from build123d import *

# Parameters (mm, degrees)
SKETCH1_W           = 18.56
SKETCH1_H           = 33.36
BOSS_EXTRUDE1_DEPTH = 1.64
FILLET1_R           = 1.2
SKETCH2_W           = 9.12
SKETCH2_H           = 5.3
CUT_EXTRUDE1_DEPTH  = 35.665510237
BOSS_EXTRUDE2_DEPTH = 6.1
SKETCH4_W           = 6.35
SKETCH4_H           = 0.5
CUT_EXTRUDE2_DEPTH  = 5
SKETCH5_W           = 6.35
SKETCH5_H           = 0.5
CUT_EXTRUDE3_DEPTH  = 0.4
SKETCH7_W           = 7
SKETCH7_H           = 7
BOSS_EXTRUDE3_DEPTH = 1.25
SKETCH8_W           = 3
SKETCH8_H           = 2.13
BOSS_EXTRUDE4_DEPTH = 1


with BuildPart() as part:
    # Sketch1 → Boss-Extrude1 (new body)
    with BuildSketch(Plane(origin=(0, 0, 0), x_dir=(1, 0, 0), z_dir=(0, 1, 0))):
        with Locations((0, -16.68)):
            Rectangle(SKETCH1_W, SKETCH1_H)
    extrude(amount=BOSS_EXTRUDE1_DEPTH)

    # Fillet1
    fillet1_edges = [part.edges().sort_by_distance(p)[0] for p in [
        (-9.28, 0.82, 0),
        (9.28, 0.82, 0),
        (9.28, 0.82, 33.36),
        (-9.28, 0.82, 33.36),
    ]]
    fillet(fillet1_edges, radius=FILLET1_R)

    # Sketch2 → Cut-Extrude1 (cut, through all)
    with BuildSketch(Plane(origin=(0, 1.64, 0), x_dir=(1, 0, 0), z_dir=(0, 1, 0))):
        with Locations((0, -2.65)):
            Rectangle(SKETCH2_W, SKETCH2_H)
    extrude(amount=-CUT_EXTRUDE1_DEPTH, mode=Mode.SUBTRACT)

    # Sketch3 → Boss-Extrude2 (add)
    with BuildSketch(Plane(origin=(0, 0, 5.3), x_dir=(-1, 0, 0), z_dir=(0, 0, -1))):
        with BuildLine():
            Line((-3.175, 0), (3.175, 0))
            ThreePointArc((3.175, 0), (4.094238816, 0.380761184), (4.475, 1.3))
            Line((4.475, 1.3), (4.475, 1.8))
            ThreePointArc((4.475, 1.8), (4.094238816, 2.719238816), (3.175, 3.1))
            Line((3.175, 3.1), (-3.175, 3.1))
            ThreePointArc((-3.175, 3.1), (-4.094238816, 2.719238816), (-4.475, 1.8))
            Line((-4.475, 1.8), (-4.475, 1.3))
            ThreePointArc((-4.475, 1.3), (-4.094238816, 0.380761184), (-3.175, 0))
        make_face()
    extrude(amount=BOSS_EXTRUDE2_DEPTH)

    # Sketch4 → Cut-Extrude2 (cut)
    with BuildSketch(Plane(origin=(0, 0, -0.8), x_dir=(-1, 0, 0), z_dir=(0, 0, -1))):
        with BuildLine():
            Line((3.175, 2.8), (-3.175, 2.8))
            ThreePointArc((-3.175, 2.8), (-3.882106781, 2.507106781), (-4.175, 1.8))
            Line((-4.175, 1.8), (-4.175, 1.3))
            ThreePointArc((-4.175, 1.3), (-3.882106781, 0.592893219), (-3.175, 0.3))
            Line((-3.175, 0.3), (3.175, 0.3))
            ThreePointArc((3.175, 0.3), (3.882106781, 0.592893219), (4.175, 1.3))
            Line((4.175, 1.3), (4.175, 1.8))
            ThreePointArc((4.175, 1.8), (3.882106781, 2.507106781), (3.175, 2.8))
        make_face()
        with Locations((0, 1.55)):
            Rectangle(SKETCH4_W, SKETCH4_H, mode=Mode.SUBTRACT)
    extrude(amount=-CUT_EXTRUDE2_DEPTH, mode=Mode.SUBTRACT)

    # Sketch5 → Cut-Extrude3 (cut)
    with BuildSketch(Plane(origin=(0, 0, -0.8), x_dir=(-1, 0, 0), z_dir=(0, 0, -1))):
        with Locations((0, 1.55)):
            Rectangle(SKETCH5_W, SKETCH5_H)
    extrude(amount=-CUT_EXTRUDE3_DEPTH, mode=Mode.SUBTRACT)

    # Sketch7 → Boss-Extrude3 (add)
    with BuildSketch(Plane(origin=(0, 1.64, 0), x_dir=(1, 0, 0), z_dir=(0, 1, 0))):
        with Locations((0, -19.07)):
            Rectangle(SKETCH7_W, SKETCH7_H)
    extrude(amount=BOSS_EXTRUDE3_DEPTH)

    # Sketch8 → Boss-Extrude4 (add)
    with BuildSketch(Plane(origin=(0, 1.64, 0), x_dir=(1, 0, 0), z_dir=(0, 1, 0))):
        with Locations((2.68, -27.945)):
            Rectangle(SKETCH8_W, SKETCH8_H)
    extrude(amount=BOSS_EXTRUDE4_DEPTH)


solid = part.part
Can you work these out from the model? Positions are in its coordinate system, mm. A direction names the side the tool comes from. Round coordinates to 2 decimals unless told otherwise and drop trailing zeros. Loops run counter-clockwise (first coordinate to the right, second up) from the corner with the lowest first, then second, coordinate; pieces in that order, holes last. Notation, with made-up numbers: (46, -18) - (84, -18) arc R24 cw to (84, -3) - close; hole circle Ø10 at (-34, -25.75). An arc over 180 degrees is marked (long way). Write item = value, one per line. Start each with the question number.
(1) For P1, Ø2, axis at x = 0.5, z = 20, coming from the +Y side; P2, Ø1, axis at x = 1.5, y = 2, coming from the -Z side; P3, Ø1.4, axis at y = 2.5, z = 19, coming from the -X side, each with a flat end and sliding along its axis, tell me the tip position at first contact or that it passes through.
(2) If I drill on probe 1 along Z at (x, y) = (1.75, 2.3); probe 2 along Y at (x, z) = (0, 1.5); probe 3 along Z at (x, y) = (2, 2.7), over which ranges is the centre line in solid material (lowest first)? Write a range as [from, to].
(3) If we section it at A-A (x = 2.5): Please give me the cut outline in (y, z).
(4) If we mould it in two halves opening along X, with no side actions, what happens to faces 5 (the face through (3.5, 2, 19)), 6 (the face through (0, 2.89, 19)), 7 (the face through (-4.084, 0.371, 2.293))? For each: released by +X, released by -X, zero draft, split by the parting line, or undercut.
(5) If we section it at B-B (z = 21.5): Please give me the cut outline in (x, y).
(6) For faces 1 (the face through (6, 1, 0)), 2 (the face through (3.89, 0.6, 1.66)), 3 (the face through (1.18, 2, 28)), 4 (the face through (4.56, 0.8, 2.7)), which set-ups out of +Z, -Z, +X, -X, +Y, -Y let a thin tool reach every point of the face, with its end or its side?
(7) If we section it at C-C (y = 0.7): Please give me the cut outline in (x, z) (3 decimals).
(8) If we section it at D-D (x = -1): Please give me the cut outline in (y, z).
Ans:
q1.P1 = 2.89
q1.P2 = -0.4
q1.P3 = -3.5
q2.probe_1 = [4.2, 5.3], [15.57, 22.57], [26.88, 29.01]
q2.probe_2 = [0, 0.3], [1.3, 1.8], [2.8, 3.1]
q2.probe_3 = [4.2, 5.3], [15.57, 22.57]
q3.outline = (0, -0.8) - (0.3, -0.8) - (0.3, 4.2) - (1.3, 4.2) - (1.3, -0.4) - (1.8, -0.4) - (1.8, 4.2) - (2.8, 4.2) - (2.8, -0.8) - (3.1, -0.8) - (3.1, 5.3) - (1.64, 5.3) - (1.64, 15.57) - (2.89, 15.57) - (2.89, 22.57) - (1.64, 22.57) - (1.64, 26.88) - (2.64, 26.88) - (2.64, 29.01) - (1.64, 29.01) - (1.64, 33.36) - (0, 33.36) - close
q4.face_5 = released by +X
q4.face_6 = zero draft
q4.face_7 = undercut
q5.outline = (-9.28, 0) - (9.28, 0) - (9.28, 1.64) - (3.5, 1.64) - (3.5, 2.89) - (-3.5, 2.89) - (-3.5, 1.64) - (-9.28, 1.64) - close
q6.face_1 = -Z, +X, +Y, -Y
q6.face_2 = -Z
q6.face_3 = +Z, -X, +Y
q6.face_4 = -Z, +Y, -Y
q7.outline = (-9.28, 1.2) arc R1.2 ccw to (-8.08, 0) - (-4.56, 0) - (-4.56, 5.3) - (-4.328, 5.3) - (-4.328, -0.8) - (-3.975, -0.8) - (-3.975, 4.2) - (3.975, 4.2) - (3.975, -0.8) - (4.328, -0.8) - (4.328, 5.3) - (4.56, 5.3) - (4.56, 0) - (8.08, 0) arc R1.2 ccw to (9.28, 1.2) - (9.28, 32.16) arc R1.2 ccw to (8.08, 33.36) - (-8.08, 33.36) arc R1.2 ccw to (-9.28, 32.16) - close
q8.outline = (0, -0.8) - (0.3, -0.8) - (0.3, 4.2) - (1.3, 4.2) - (1.3, -0.4) - (1.8, -0.4) - (1.8, 4.2) - (2.8, 4.2) - (2.8, -0.8) - (3.1, -0.8) - (3.1, 5.3) - (1.64, 5.3) - (1.64, 15.57) - (2.89, 15.57) - (2.89, 22.57) - (1.64, 22.57) - (1.64, 33.36) - (0, 33.36) - close
